Here's how the part is built. I have some questions about the finished solid (model axes, mm). Face numbers are marked on the shaded views. Round coordinates to 2 decimals unless told otherwise and drop trailing zeros. Loops run counter-clockwise (first coordinate to the right, second up) from the corner with the lowest first, then second, coordinate; pieces in that order, holes last. Notation, with made-up numbers: (24.25, -28.75) - (80.25, -28.75) arc R13 ccw to (80.25, -7.75) - close; hole circle Ø9 at (7.5, 23). An arc over 180 degrees is marked (long way). Answer as a JSON object with one key per item and string values. Group by question number.
1) If we mould it in two halves opening along X, with no side actions, what happens to the marked faces 1, 2 and 3? For each: pulls with the +X half, pulls with the -X half, needs draft (parallel to the pull), parting line crosses it, or undercut.
2) I want a section at C-C, the plane z = 6.5. Please give me the cut outline in (x, y), then the cut area to 3 significant figures.
3) Will these pins go through, and if not, where does the flat tip stop? P1, Ø3, axis at y = -52.5, z = 8, coming from the +X side; P2, Ø5, axis at y = -210.5, z = 3.5, coming from the +X side; P3, Ø4, axis at y = -48.5, z = 4, coming from the -X side.
4) If I drill on line 1 along X through (y, z) = (-55.5, 2); line 2 along X through (y, z) = (-159.5, 5.75); line 3 along X through (y, z) = (-182, 0.5), over which ranges is the centre line in solid material (lowest first)? Write a range as [from, to].
5) I want a section at A-A, the plane y = -184. Please give me the cut outline in (x, z).
6) I want a section at B-B, the plane x = -19.5. Please give me the cut outline in (y, z).
7) I want a section at D-D, the plane y = -84.5. Please give me the cut outline in (x, z), then the cut area to 3 significant figures.
from build123d import *

# Parameters (mm, degrees)
SKETCH1_R           = 3
BOSS_EXTRUDE2_DEPTH = 10
FILLET1_R           = 20
FILLET2_R           = 20
CUT_EXTRUDE1_START  = -10
CUT_EXTRUDE1_DEPTH  = 10
FILLET3_R           = 5
CUT_EXTRUDE6_DEPTH  = 10
SKETCH7_W           = 65.010384479
SKETCH7_H           = 38.033760717
CUT_EXTRUDE7_DEPTH  = 10


with BuildPart() as part:
    # Sketch1 → Boss-Extrude2 (new body)
    with BuildSketch(Plane.XY):
        with BuildLine():
            Line((-30, 15.770412854), (-30, 0))
            Line((-30, 0), (-17.5, -210))
            ThreePointArc((-17.5, -210), (0, -227.5), (17.5, -210))
            Line((17.5, -210), (30, 0))
            Line((30, 0), (30, 15.770412854))
            Line((30, 15.770412854), (-30, 15.770412854))
        make_face()
        with Locations((-15, 0)):
            Circle(SKETCH1_R, mode=Mode.SUBTRACT)
        with Locations((15, 0)):
            Circle(SKETCH1_R, mode=Mode.SUBTRACT)
        Polygon((0, -205), (6, -205), (6, -215), (-6, -215), (-6, -205), align=None, mode=Mode.SUBTRACT)
    extrude(amount=BOSS_EXTRUDE2_DEPTH)

    # Fillet1
    fillet1_edges = [part.edges().sort_by_distance(p)[0] for p in [
        (-30, 15.770412854, 5),
    ]]
    fillet(fillet1_edges, radius=FILLET1_R)

    # Fillet2
    fillet2_edges = [part.edges().sort_by_distance(p)[0] for p in [
        (30, 15.770412854, 5),
    ]]
    fillet(fillet2_edges, radius=FILLET2_R)

    # Sketch4 → Cut-Extrude1 (cut)
    with BuildSketch(Plane.XY.offset(10).offset(CUT_EXTRUDE1_START)):
        Polygon((-15.651797422, -15), (0.190220551, -102.160979768), (15.643622882, -15), (15, -15), align=None)
        Polygon((-22.473027071, -25.6531452), (-13.367328465, -178.628881795), (-4.134156204, -126.551525408), align=None)
        Polygon((22.230419841, -27.161313899), (4.615986353, -126.511039477), (13.430162671, -175.005634359), align=None)
        with BuildLine():
            Line((0.291609598, -150.901585116), (-7.372445375, -194.128735111))
            ThreePointArc((-7.372445375, -194.128735111), (0.476576628, -192.506490497), (8.225632191, -194.553674383))
            Line((8.225632191, -194.553674383), (0.291609598, -150.901585116))
        make_face()
    extrude(amount=CUT_EXTRUDE1_DEPTH, mode=Mode.SUBTRACT)

    # Fillet3
    fillet3_edges = [part.edges().sort_by_distance(p)[0] for p in [
        (8.225632191, -194.553674383, 5),
        (-7.372445375, -194.128735111, 5),
        (-15.651797422, -15, 5),
        (15.643622882, -15, 5),
    ]]
    fillet(fillet3_edges, radius=FILLET3_R)

    # Sketch5 → Cut-Extrude6 (cut)
    with BuildSketch(Plane.XY.offset(10)):
        with BuildLine():
            Line((29.260488635, 0), (20, 0))
            Line((20, 0), (20, -20))
            Line((20, -20), (28.80952381, -20))
            Line((28.80952381, -20), (29.677502384, -5.417959945))
            ThreePointArc((29.677502384, -5.417959945), (29.653859351, -2.694751229), (29.260488635, 0))
        make_face()
        with BuildLine():
            Line((20, 12.921923742), (20, 0))
            Line((20, 0), (29.260488635, 0))
            ThreePointArc((29.260488635, 0), (25.96931496, 7.420606017), (20, 12.921923742))
        make_face()
    extrude(amount=-CUT_EXTRUDE6_DEPTH, mode=Mode.SUBTRACT)

    # Sketch7 → Cut-Extrude7 (cut)
    with BuildSketch(Plane.XY.offset(10)):
        with Locations((-3.695668429, -0.983119642)):
            Rectangle(SKETCH7_W, SKETCH7_H)
    extrude(amount=-CUT_EXTRUDE7_DEPTH, mode=Mode.SUBTRACT)


solid = part.part
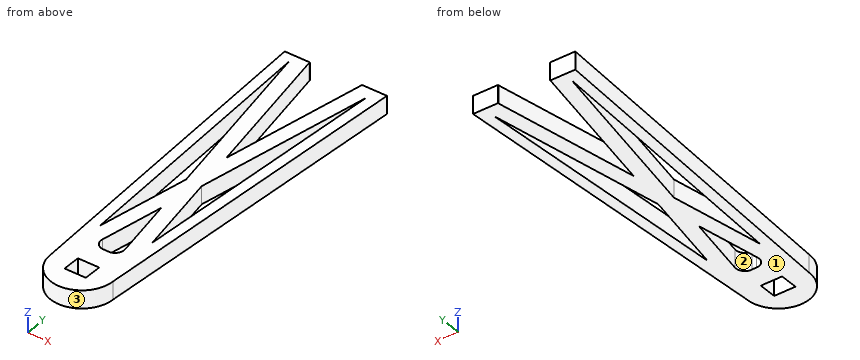
Outcome:
{
 "1": {"face 1": "needs draft", "face 2": "undercut", "face 3": "parting line crosses it"},
 "2": {"outline": "(-28.81, -20) - (-17.5, -210) arc R17.5 ccw to (17.5, -210) - (28.81, -20) - (14.68, -20) arc R5 cw to (14.6, -20.87) - (0.19, -102.16) - (-14.58, -20.89) arc R5 cw to (-14.66, -20) - close; hole (-22.47, -25.65) - (-13.37, -178.63) - (-4.13, -126.55) - close; hole (-6.05, -186.66) arc R5 ccw to (-0.87, -192.52) arc R17.5 cw to (1.46, -192.56) arc R5 ccw to (6.8, -186.68) - (0.29, -150.9) - close; hole (-6, -215) - (6, -215) - (6, -205) - (-6, -205) - close; hole (4.62, -126.51) - (13.43, -175.01) - (22.23, -27.16) - close", "area": "5,840 mm^2"},
 "3": {"P1": "x = 26.96", "P2": "x = 17.62", "P3": "x = -27.23"},
 "4": {"line 1": "[-26.7, -20.7], [-17.05, -8.29], [8.46, 17.21], [20.54, 26.7]", "line 2": "[-20.51, -14.51], [-9.98, -1.23], [1.85, 10.61], [14.35, 20.51]", "line 3": "[-19.17, -5.22], [5.94, 19.17]"},
 "5": {"outline": "(-19.05, 0) - (-5.58, 0) - (-5.58, 10) - (-19.05, 10) - close; (6.31, 0) - (19.05, 0) - (19.05, 10) - (6.31, 10) - close"},
 "6": {"outline": "(-176.4, 0) - (-75.6, 0) - (-75.6, 10) - (-176.4, 10) - close; (-42.01, 0) - (-20, 0) - (-20, 10) - (-42.01, 10) - close"},
 "7": {"outline": "(-24.97, 0) - (-18.97, 0) - (-18.97, 10) - (-24.97, 10) - close; (-11.78, 0) - (-3.02, 0) - (-3.02, 10) - (-11.78, 10) - close; (3.32, 0) - (12.06, 0) - (12.06, 10) - (3.32, 10) - close; (18.82, 0) - (24.97, 0) - (24.97, 10) - (18.82, 10) - close", "area": "297 mm^2"}
}
